from build123d import *

# Parameters (mm, degrees)
F1_DEPTH = 7.5
F2_R     = 2.5
F3_DEPTH = 2
F4_R     = 5
F5_R     = 3
F6_R     = 3
F7_R     = 5
F8_R     = 1.999


# Not quite as in the source:
# - a fillet or chamfer is up to 0.001 mm smaller than in the source, because OpenCascade refuses the exact size


with BuildPart() as f1:
    # F0 (on Right) → F1 (new body, symmetric)
    with BuildSketch(Plane.YZ):
        Polygon((-58.3, 0), (-88.3, 0), (-88.2997653641, -2), (-56.8037653641, -2), (-46.5037653641, 33), (0, 33), (46.5037653641, 33), (56.8037653641, -2), (88.2997653641, -2), (88.3, 0), (58.3, 0), (48, 35), (0, 35), (-48, 35), align=None)
    extrude(amount=F1_DEPTH, both=True)

    # F2 (on face) → F3 (cut)
    with BuildSketch(Plane.XY.offset(35)):
        with Locations((0, -24)):
            Circle(F2_R)
        with Locations((0, 24)):
            Circle(F2_R)
    extrude(amount=-F3_DEPTH, mode=Mode.SUBTRACT)

    # F4
    f4_edges = [f1.edges().sort_by_distance(p)[0] for p in [
        (0, -56.803765, -2),
    ]]
    fillet(f4_edges, radius=F4_R)

    # F5
    f5_edges = [f1.edges().sort_by_distance(p)[0] for p in [
        (0, -58.3, 0),
    ]]
    fillet(f5_edges, radius=F5_R)

    # F6
    f6_edges = [f1.edges().sort_by_distance(p)[0] for p in [
        (0, 58.3, 0),
    ]]
    fillet(f6_edges, radius=F6_R)

    # F7
    f7_edges = [f1.edges().sort_by_distance(p)[0] for p in [
        (0, 56.803765, -2),
    ]]
    fillet(f7_edges, radius=F7_R)

    # F8 (radius 2 in the source; OpenCascade refuses exactly that, so slightly less here)
    f8_edges = [f1.edges().sort_by_distance(p)[0] for p in [
        (0, -88.3, 0),
        (0, 88.3, 0),
    ]]
    fillet(f8_edges, radius=F8_R)


solid = f1.part
Could you check a few things on this model? Use its own coordinates, in mm. A direction names the side the tool comes from. Give positions to 0.01 mm unless a question says otherwise; leave off trailing zeros. Order: outer loops, then holes, each group sorted by start corner. A loop starts at its lowest first (then second) coordinate and runs counter-clockwise, first axis right, second up.
1. Will this pin go through, and if not, where does the flat tip stop? P1, Ø7.5, axis at x = -1.5, y = -69.5, coming from the +Z side.
2. Suppose I cut it at A-A (x = 0). Give the number of separate pieces and of enclosed holes in the cut face, plus the area to 3 significant figures.
3. I need wall thicknesses on L1, parallel to Y at x = 0, z = 34.3; L2, parallel to Y at x = 0, z = 34.15; L3, parallel to Z at x = -5.5, y = 21. Which ranges of each line are inside material? Lowest first, please.
4. For faces 4 (the flat face through (0, 74, 0)), 5 (the flat face through (0.11, -51.19, 17.07)), 6 (the flat face through (0, -73, 0)), which set-ups out of +Z, -Z, +X, -X, +Y, -Y let a thin tool reach every point of the face, with its end or its side?
5. Suppose I cut it at B-B (y = -24). List the corners of the cut face in (x, z) for me.
6. Suppose I cut it at C-C (z = 25). List the corners of the cut face in (x, y) for me, plus the area to 3 significant figures.
7. We'd pull the mould along Y, two halves only. Please class faces 1 (the flat face through (0.11, 52.9, 18.35)), 2 (the flat face through (0, 1, 35)), 3 (the flat face through (0.105, 51.061, 17.514)): pulls with the +Y half, pulls with the -Y half, needs draft (parallel to the pull), parting line crosses it, or undercut.
Solved:
1. P1: stops at z = 0
2. separate pieces: 3
2. enclosed holes: 0
2. area: 433 mm2
3. L1: y = -48.21 to -26.5, -21.5 to 21.5, 26.5 to 48.21
3. L2: y = -48.25 to -26.5, -21.5 to 21.5, 26.5 to 48.25
3. L3: z = 33 to 35
4. face 4: +Z, +X, -X, +Y
4. face 5: -Z, +X, -X
4. face 6: +Z, +X, -X, -Y
5. outline: (-7.5, 33) - (-2.5, 33) - (-2.5, 35) - (-7.5, 35) - close; (2.5, 33) - (7.5, 33) - (7.5, 35) - (2.5, 35) - close
6. outline: (-7.5, -50.94) - (7.5, -50.94) - (7.5, -48.86) - (-7.5, -48.86) - close; (-7.5, 48.86) - (7.5, 48.86) - (7.5, 50.94) - (-7.5, 50.94) - close
6. area: 62.5 mm2
7. face 1: pulls with the +Y half
7. face 2: needs draft
7. face 3: undercut
